```python
from build123d import *

# Parameters (mm, degrees)
PAD_DEPTH       = 2
SKETCH010_W     = 86
SKETCH010_H     = 2
PAD001_DEPTH    = 55
SKETCH009_R     = 1.4
POCKET_DEPTH    = 2
SKETCH003_W     = 15
SKETCH003_H     = 20
PAD002_DEPTH    = 6.85
SKETCH004_R     = 1.4
POCKET001_DEPTH = 15
SKETCH005_R     = 1.4
POCKET002_DEPTH = 15
SKETCH006_W     = 5
SKETCH006_H     = 5
PAD003_DEPTH    = 5
SKETCH007_R     = 1.4
POCKET003_DEPTH = 5
SKETCH008_R     = 1.4
POCKET004_DEPTH = 5


with BuildPart() as part:
    # Sketch → Pad (new body)
    with BuildSketch(Plane.XY):
        with BuildLine():
            Line((-43, 2), (43, 2))
            Line((43, 2), (43, -23))
            ThreePointArc((41, -25), (42.414214, -24.414214), (43, -23))
            Line((41, -25), (-41, -25))
            ThreePointArc((-43, -23), (-42.414214, -24.414214), (-41, -25))
            Line((-43, -23), (-43, 2))
        make_face()
    extrude(amount=PAD_DEPTH)

    # Sketch010 (on Face8 of Pad) → Pad001 (join)
    with BuildSketch(Plane.XY.offset(2)):
        with Locations((0, 1)):
            Rectangle(SKETCH010_W, SKETCH010_H)
    extrude(amount=PAD001_DEPTH)

    # Sketch009 (on Face13 of Pad001) → Pocket (cut)
    with BuildSketch(Plane.XZ):
        with Locations((-7.5, 52.5)):
            Circle(SKETCH009_R)
        with Locations((7.5, 52.5)):
            Circle(SKETCH009_R)
    extrude(amount=-POCKET_DEPTH, mode=Mode.SUBTRACT)

    # Sketch003 (on Face7 of Pocket) → Pad002 (join)
    with BuildSketch(Plane.XY.offset(2)):
        with Locations((-23.5, -10)):
            Rectangle(SKETCH003_W, SKETCH003_H)
        with Locations((23.5, -10)):
            Rectangle(SKETCH003_W, SKETCH003_H)
    extrude(amount=PAD002_DEPTH)

    # Sketch004 (on Face16 of Pad002) → Pocket001 (cut)
    with BuildSketch(Plane(origin=(-31, 0, 0), x_dir=(0, -1, 0), z_dir=(-1, 0, 0))):
        with Locations((5, 5)):
            Circle(SKETCH004_R)
        with Locations((15, 5)):
            Circle(SKETCH004_R)
    extrude(amount=-POCKET001_DEPTH, mode=Mode.SUBTRACT)

    # Sketch005 (on Face21 of Pocket001) → Pocket002 (cut)
    with BuildSketch(Plane.YZ.offset(31)):
        with Locations((-15, 5)):
            Circle(SKETCH005_R)
        with Locations((-5, 5)):
            Circle(SKETCH005_R)
    extrude(amount=-POCKET002_DEPTH, mode=Mode.SUBTRACT)

    # Sketch006 (on Face7 of Pocket002) → Pad003 (join)
    with BuildSketch(Plane.XY.offset(2)):
        with Locations((-7.5, -17.5)):
            Rectangle(SKETCH006_W, SKETCH006_H)
        with Locations((7.5, -17.5)):
            Rectangle(SKETCH006_W, SKETCH006_H)
    extrude(amount=PAD003_DEPTH)

    # Sketch007 (on Face23 of Pad003) → Pocket003 (cut)
    with BuildSketch(Plane.XZ.offset(20)):
        with Locations((-7.5, 4.5)):
            Circle(SKETCH007_R)
    extrude(amount=-POCKET003_DEPTH, mode=Mode.SUBTRACT)

    # Sketch008 (on Face27 of Pocket003) → Pocket004 (cut)
    with BuildSketch(Plane.XZ.offset(20)):
        with Locations((7.5, 4.5)):
            Circle(SKETCH008_R)
    extrude(amount=-POCKET004_DEPTH, mode=Mode.SUBTRACT)


solid = part.part
```
For this review, take the finished solid that the model builds, in its own axes (mm). A direction names the side the tool comes from. Coordinates: 2 decimals unless noted, no trailing zeros. Order: outer loops, then holes, each group sorted by start corner. A loop starts at its lowest first (then second) coordinate and runs counter-clockwise, first axis right, second up. Notation, with made-up numbers: (-39.5, 5.25) - (11.5, 5.25) arc R16 ccw to (11.5, 13.25) - close; hole circle Ø10 at (63.25, 65). An arc over 180 degrees is marked (long way). Answer as a JSON object with one key per item and string values. Group by question number.
1. Clearance check with flat-ended pins moving along their axes: P1, Ø3, axis at y = -15, z = 5, coming from the -X side; P2, Ø5.5, axis at y = -7, z = 4.5, coming from the +X side; P3, Ø2, axis at y = -15, z = 5, coming from the +X side; P4, Ø3, axis at x = -23, y = -16.5, coming from the +Z side. State where each tip first meets the part, or that it passes through.
2. The part is to be moulded in two halves that separate along Y. For faces 1 (the cylindrical face through (23.605, -3.665, 5.421)), 2 (the flat face through (-31, -10, 5)), 3 (the flat face through (-1, 2, 28)), say which applies: pulls with the +Y half, pulls with the -Y half, needs draft (parallel to the pull), parting line crosses it, or undercut.
3. For faces 4 (the cylindrical face through (6.1, -17.54, 4.56)), 5 (the flat face through (-24, -20, 5)), 6 (the cylindrical face through (-23.6, -13.97, 5.95)), 7 (the flat face through (31, -10, 5)), 8 (the flat face through (10, -18, 4)), list the 3-axis set-ups (+Z, -Z, +X, -X, +Y, -Y) from which the entire face can be reached by the end or side of a thin tool; tool diameter is ignored.
4. We need section C-C on x = -25.5. State the section outline as (y, z) points.
5. We need section D-D on z = 24.5. State the section outline as (x, y) points.
6. We need section A-A on y = -5. State the section outline as (x, z) points.
7. We need section B-B on x = 7.5. State the section outline as (y, z) points.
8. For probe 1 along Z at (x, y) = (7.5, -17.85); probe 2 along X at (y, z) = (-2, 8.5); probe 3 along X at (y, z) = (-16.75, 5), list the stretches that pass through material, from the lowest coordinate up.
Final values:
{
 "1": {"P1": "x = -31", "P2": "x = 43", "P3": "x = 10", "P4": "z = 8.85"},
 "2": {"face 1": "undercut", "face 2": "needs draft", "face 3": "pulls with the +Y half"},
 "3": {"face 4": "-Y", "face 5": "+Z, +X, -X, -Y", "face 6": "-X", "face 7": "+Z, +X, -Y", "face 8": "+Z, -Y"},
 "4": {"outline": "(-25, 0) - (2, 0) - (2, 57) - (0, 57) - (0, 8.85) - (-20, 8.85) - (-20, 2) - (-25, 2) - close; hole circle Ø2.8 at (-15, 5); hole circle Ø2.8 at (-5, 5)"},
 "5": {"outline": "(-43, 0) - (43, 0) - (43, 2) - (-43, 2) - close"},
 "6": {"outline": "(-43, 0) - (43, 0) - (43, 2) - (31, 2) - (31, 3.6) - (16, 3.6) - (16, 2) - (-16, 2) - (-16, 3.6) - (-31, 3.6) - (-31, 2) - (-43, 2) - close; (-31, 6.4) - (-16, 6.4) - (-16, 8.85) - (-31, 8.85) - close; (16, 6.4) - (31, 6.4) - (31, 8.85) - (16, 8.85) - close"},
 "7": {"outline": "(-25, 0) - (2, 0) - (2, 51.1) - (0, 51.1) - (0, 2) - (-15, 2) - (-15, 3.1) - (-20, 3.1) - (-20, 2) - (-25, 2) - close; (-20, 5.9) - (-15, 5.9) - (-15, 7) - (-20, 7) - close; (0, 53.9) - (2, 53.9) - (2, 57) - (0, 57) - close"},
 "8": {"probe 1": "0 to 3.1, 5.9 to 7", "probe 2": "-31 to -16, 16 to 31", "probe 3": "-31 to -16, -10 to -8.81, -6.19 to -5, 5 to 6.19, 8.81 to 10, 16 to 31"}
}
